Part print with two shaded views. Sizes in mm from the minimum x, y, z corner. A direction names the side the tool comes from. Round coordinates to 2 decimals unless told otherwise and drop trailing zeros. Loops run counter-clockwise (first coordinate to the right, second up) from the corner with the lowest first, then second, coordinate; pieces in that order, holes last. Notation, with made-up numbers: M 37,42.5 L 80,42.5 A20 ccw 80,64.5 Z; hole C -2.75,43.5 d6. An arc over 180 degrees is marked long. Use a Markdown table: item, result. Add a question column.
Item 1: Saw through at B-B on z = 96.5. Write the cut outline in (x, y), then the cut area to 3 significant figures.
Item 2: Tool access for the marked faces 1, 2 and 3: list every direction of +Z, -Z, +X, -X, +Y, -Y with a clear straight run to the whole face (end or side of a thin tool).
Item 3: Saw through at A-A on x = 15. Write the cut outline in (y, z).
Item 4: Wall check: L1, parallel to Z at x = 22, y = 3; L2, parallel to Z at x = 31.5, y = 24. Give the ranges that are in metal, low to high. Write a range as from..to.
Item 5: Pin check, flat tips, straight feed: P1, Ø3, axis at x = 6.5, z = 92, coming from the +Y side; P2, Ø1.5, axis at x = 31.5, y = 7, coming from the +Z side; P3, Ø6.5, axis at x = 13, z = 101.5, coming from the +Y side. Stop position of each tip, or through.
Item 6: Saw through at C-C on y = 25.5. Write the cut outline in (x, z).
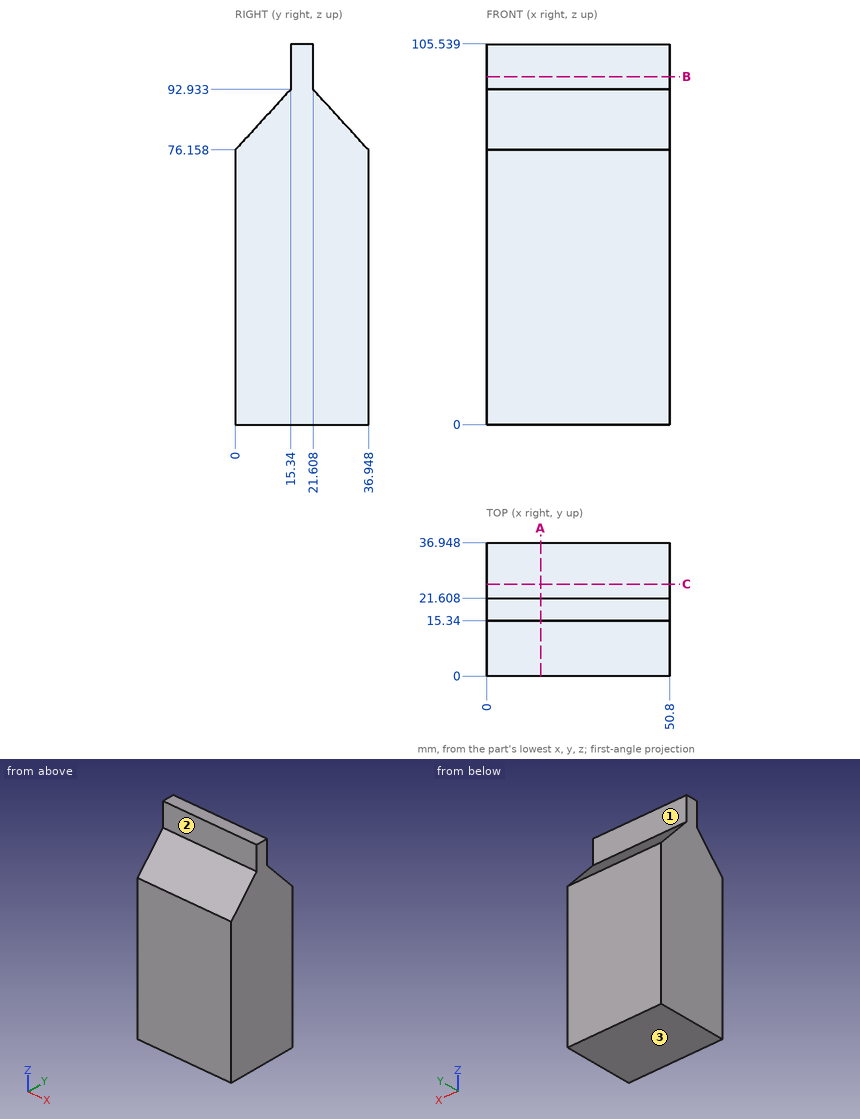
Entries:
| question | item | result |
|---|---|---|
| 1 | outline | M 0,15.34 L 50.8,15.34 L 50.8,21.61 L 0,21.61 Z |
| 1 | area | 318 mm2 |
| 2 | face 1 | +Z, +X, -X, +Y |
| 2 | face 2 | +Z, +X, -X, -Y |
| 2 | face 3 | -Z, +X, -X, +Y, -Y |
| 3 | outline | M 0,0 L 36.95,0 L 36.95,76.16 L 21.61,92.93 L 21.61,105.54 L 15.34,105.54 L 15.34,92.93 L 0,76.16 Z |
| 4 | L1 | 0..79.44 |
| 4 | L2 | 0..90.32 |
| 5 | P1 | y = 23.83 |
| 5 | P2 | z = 84.63 |
| 5 | P3 | y = 21.61 |
| 6 | outline | M 0,0 L 50.8,0 L 50.8,88.68 L 0,88.68 Z |
